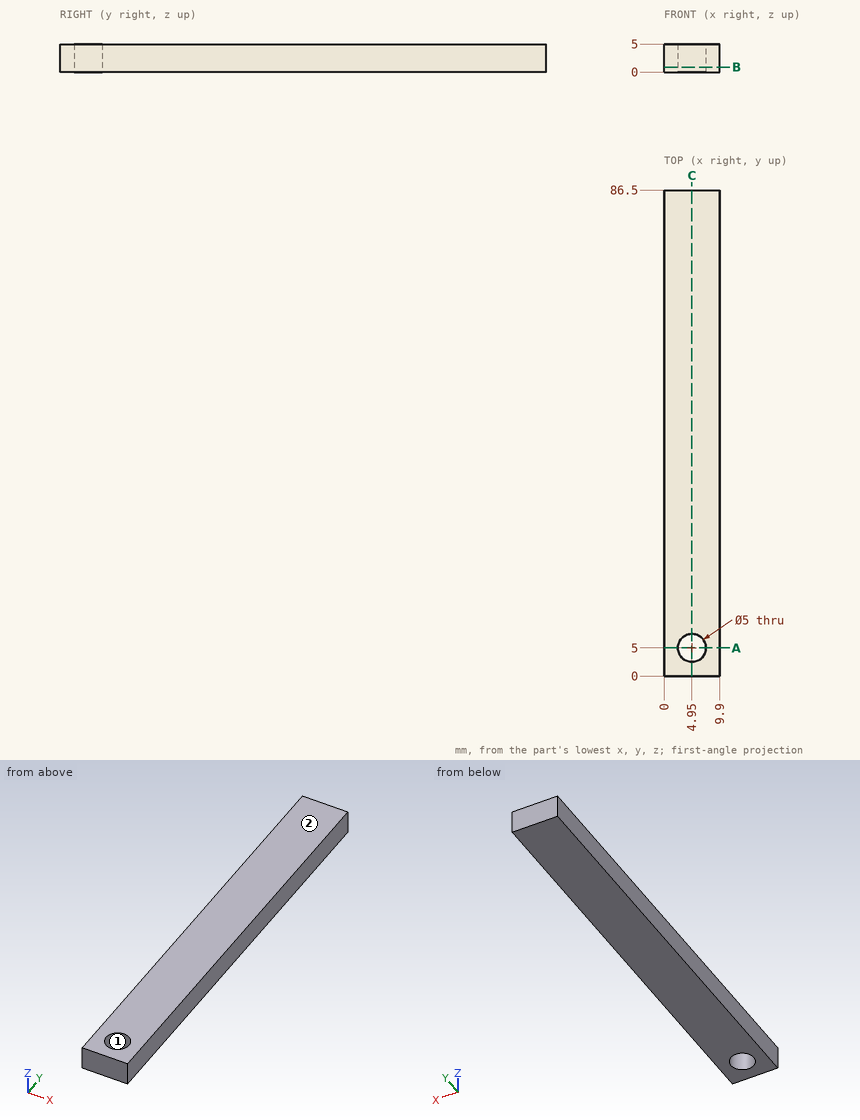
Here's the drawing with two shaded views (mm, measured from the low corner). I have some questions. Coordinates: 2 decimals unless noted, no trailing zeros. Loops run counter-clockwise (first coordinate to the right, second up) from the corner with the lowest first, then second, coordinate; pieces in that order, holes last. Notation, with made-up numbers: M 33.25,88 L 57.25,88 A19 cw 57.25,110 Z; hole C 86,-9.5 d4. An arc over 180 degrees is marked long. Put each result on its own line as item: value. Start each with the question number.
(1) Imagine slicing it at B-B on z = 0.9. List the corners of the cut face in (x, y) for me.
(2) Imagine slicing it at C-C on x = 4.95. List the corners of the cut face in (y, z) for me.
(3) Will these pins go through, and if not, where does the flat tip stop? pin 1 Ø4 at (x, y) = (4.95, 5) entering from +Z; pin 2 Ø1.5 at (x, z) = (1.5, 1) entering from -Y.
(4) We'd pull the mould along X, two halves only. Please class the marked faces 1 and 2: +X half, -X half, draft (parallel to the pull), parting line (faces both ways), or undercut.
(5) I need wall thicknesses on probe 1 along X at (y, z) = (5, 2.2); probe 2 along Y at (x, z) = (5.25, 0.5); probe 3 along Y at (x, z) = (7, 3). Which ranges of each line are inside material? Lowest first, please.
(6) Imagine slicing it at A-A on y = 5. List the corners of the cut face in (x, z) for me, and give its area (3 significant figures).
Worked answers:
1. outline: M 0,0 L 9.9,0 L 9.9,86.5 L 0,86.5 Z; hole C 4.95,5 d5
2. outline: M 0,0 L 2.5,0 L 2.5,5 L 0,5 Z; M 7.5,0 L 86.5,0 L 86.5,5 L 7.5,5 Z
3. pin 1: passes through
3. pin 2: stops at y = 0
4. face 1: undercut
4. face 2: draft
5. probe 1: x = 0 to 2.45, 7.45 to 9.9
5. probe 2: y = 0 to 2.52, 7.48 to 86.5
5. probe 3: y = 0 to 3.57, 6.43 to 86.5
6. outline: M 0,0 L 2.45,0 L 2.45,5 L 0,5 Z; M 7.45,0 L 9.9,0 L 9.9,5 L 7.45,5 Z
6. area: 24.5 mm2
